Check sheet for the modelled part. Datum: model origin and axes. Units: mm. Face numbers are marked on the shaded views. A direction names the side the tool comes from. Coordinates: 2 decimals unless noted, no trailing zeros. Write each loop counter-clockwise with the first axis right and the second up, starting at its lowest first coordinate (ties: lowest second). Pieces come first, ordered by that corner, then holes. Notation, with made-up numbers: (47.5, 19.5) -> (53.5, 19.5) arc R30 cw to (53.5, 51.5) -> close; hole circle Ø8 at (20, -27.5). An arc over 180 degrees is marked (long way). One line per item, written item: value. Start each with the question number.
1) Sectioned sample at A-A on y = 50.8. Enter the section's corners in (x, z) (3 decimals).
2) Gauge pin test, flat ends, axial feed: P1, Ø2, axis at x = 43, y = 84.5, coming from the +Z side (3 decimals); P2, Ø2, axis at y = 31.5, z = 166.5, coming from the -X side (3 decimals); P3, Ø4, axis at y = 47, z = 102.5, coming from the +X side. Record the tip position at first contact, or that the pin passes through.
3) Draft check along Z on the marked faces 4, 5, 6 and 7. Enter one of: +Z half, -Z half, draft (parallel to the pull), parting line (faces both ways), or undercut.
4) Sectioned sample at D-D on z = 24. Enter the section's corners in (x, y) (3 decimals), plus the area to 3 significant figures.
5) Scan lines: line 1 along Z through (x, y) = (10, 38) (3 decimals); line 2 along X through (y, z) = (5.5, 161) (3 decimals); line 3 along Z through (x, y) = (122.5, 58) (3 decimals). Record each from-to range of solid material in increasing order. Write a range as [from, to].
6) Set-up check for the marked faces 1, 2 and 3: record each of +Z, -Z, +X, -X, +Y, -Y from which the full face is reachable in a straight line by a thin tool's end or side.
7) Sectioned sample at B-B on x = 36. Enter the section's corners in (y, z) (3 decimals).
8) Sectioned sample at C-C on y = 8.5. Enter the section's corners in (x, z) (3 decimals).
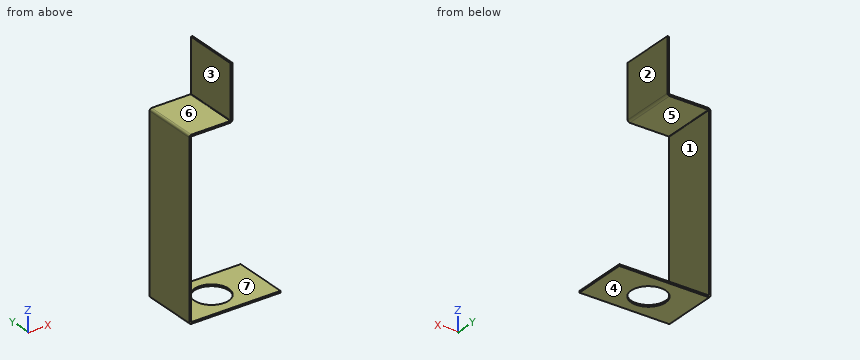
```python
from build123d import *

# Parameters (mm, degrees)
BASE_FLANGE1_DEPTH = 101.6
SKETCH6_R          = 31.75
CUT_EXTRUDE1_DEPTH = 462.763337653


# Sheet-metal steps are written as plain solids
with BuildPart() as part:
    # Sketch1 → Base-Flange1 (new body)
    with BuildSketch(Plane(origin=(0, 0, 0), x_dir=(1, 0, 0), z_dir=(0, 1, 0))):
        with BuildLine():
            Line((76.2, -228.6), (76.2, -130.9116))
            ThreePointArc((76.2, -130.9116), (75.054318885, -128.145681115), (72.2884, -127))
            Line((72.2884, -127), (0.7366, -127))
            ThreePointArc((0.7366, -127), (0.215745145, -126.784254855), (0, -126.2634))
            Line((0, -126.2634), (0, 0))
            Line((0, 0), (0, 189.7634))
            ThreePointArc((0, 189.7634), (0.215745145, 190.284254855), (0.7366, 190.5))
            Line((0.7366, 190.5), (165.1, 190.5))
            Line((165.1, 190.5), (165.1, 193.675))
            Line((165.1, 193.675), (0.7366, 193.675))
            ThreePointArc((0.7366, 193.675), (-2.029318885, 192.529318885), (-3.175, 189.7634))
            Line((-3.175, 189.7634), (-3.175, 0))
            Line((-3.175, 0), (-3.175, -126.2634))
            ThreePointArc((-3.175, -126.2634), (-2.029318885, -129.029318885), (0.7366, -130.175))
            Line((0.7366, -130.175), (72.2884, -130.175))
            ThreePointArc((72.2884, -130.175), (72.809254855, -130.390745145), (73.025, -130.9116))
            Line((73.025, -130.9116), (73.025, -228.6))
            Line((73.025, -228.6), (76.2, -228.6))
        make_face()
    extrude(amount=BASE_FLANGE1_DEPTH)

    # Sketch6 → Cut-Extrude1 (cut, through all)
    with BuildSketch(Plane.XY.offset(-190.5)):
        with Locations((74.5998, 50.8)):
            Circle(SKETCH6_R)
    extrude(amount=-CUT_EXTRUDE1_DEPTH, mode=Mode.SUBTRACT)


solid = part.part
```
Answers:
1. outline: (-3.175, -189.763) arc R3.912 ccw to (0.737, -193.675) -> (42.85, -193.675) -> (42.85, -190.5) -> (0.737, -190.5) arc R0.737 cw to (0, -189.763) -> (0, 126.263) arc R0.737 cw to (0.737, 127) -> (72.288, 127) arc R3.912 ccw to (76.2, 130.912) -> (76.2, 228.6) -> (73.025, 228.6) -> (73.025, 130.912) arc R0.737 cw to (72.288, 130.175) -> (0.737, 130.175) arc R3.912 ccw to (-3.175, 126.263) -> close; (106.35, -193.675) -> (165.1, -193.675) -> (165.1, -190.5) -> (106.35, -190.5) -> close
2. P1: stops at z = 130.175
2. P2: stops at x = 73.025
2. P3: stops at x = 0
3. face 4: -Z half
3. face 5: undercut
3. face 6: +Z half
3. face 7: undercut
4. outline: (-3.175, 0) -> (0, 0) -> (0, 101.6) -> (-3.175, 101.6) -> close
4. area: 323 mm2
5. line 1: z = [-193.675, -190.5], [127, 130.175]
5. line 2: x = [73.025, 76.2]
5. line 3: z = [-193.675, -190.5]
6. face 1: +X, +Y, -Y
6. face 2: +Z, +X, +Y, -Y
6. face 3: +Z, -X, +Y, -Y
7. outline: (0, -193.675) -> (101.6, -193.675) -> (101.6, -190.5) -> (0, -190.5) -> close; (0, 127) -> (101.6, 127) -> (101.6, 130.175) -> (0, 130.175) -> close
8. outline: (-3.175, -189.763) arc R3.912 ccw to (0.737, -193.675) -> (165.1, -193.675) -> (165.1, -190.5) -> (0.737, -190.5) arc R0.737 cw to (0, -189.763) -> (0, 126.263) arc R0.737 cw to (0.737, 127) -> (72.288, 127) arc R3.912 ccw to (76.2, 130.912) -> (76.2, 228.6) -> (73.025, 228.6) -> (73.025, 130.912) arc R0.737 cw to (72.288, 130.175) -> (0.737, 130.175) arc R3.912 ccw to (-3.175, 126.263) -> close
